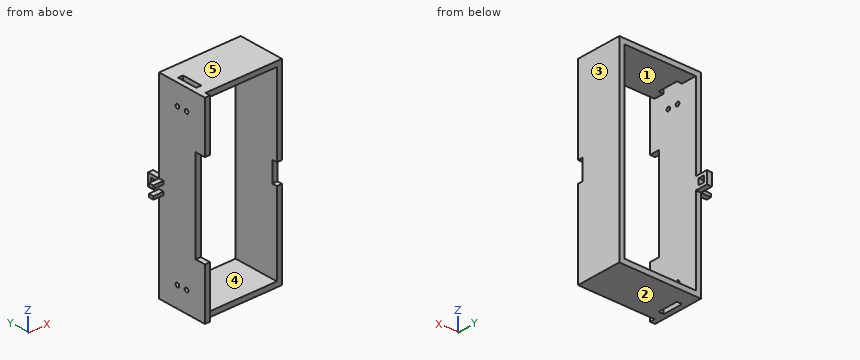
Autodesk Inventor part; units mm, degrees
ref_plane "YZ Plane" through (0, 0, 0) normal (1, 0, 0) x (0, 1, 0)
ref_plane "XZ Plane" through (0, 0, 0) normal (0, 1, 0) x (-1, 0, 0)
ref_plane "XY Plane" through (0, 0, 0) normal (0, 0, 1) x (1, 0, 0)
sketch "Sketch1" plane through (0, 0, 0) normal (1, 0, 0) x (0, 1, 0)
  line L0 (0, 0) -> (50, 0)
  line L1 (50, 0) -> (50, -50)
  line L2 (0, 0) -> (10, 0)
  line L3 (10, -50) -> (0, -50)
  line L4 (0, -50) -> (0, 0)
  line L5 (50, -50) -> (50, -190)
  line L6 (50, -190) -> (0, -190)
  line L7 (0, -190) -> (0, -140)
  line L8 (0, -140) -> (10, -140)
  line L9 (10, -140) -> (10, -50)
  line L10 (0, -105) -> (50, -105) construction
  line L11 (50, -89) -> (62, -89)
  line L12 (62, -89) -> (62, -101)
  line L13 (62, -101) -> (50, -101)
  line L14 (50, -101) -> (50, -89)
  line L15 (59, -92) -> (53, -92)
  line L16 (53, -92) -> (53, -98)
  line L17 (53, -98) -> (59, -98)
  line L18 (59, -98) -> (59, -92)
  point P0 (50, -101)
  dimension "d0" = 50
  dimension "d4" = 50
  dimension "d5" = 10
  dimension "d8" = 190
  dimension "d9" = 50
  dimension "d10" = 12
  dimension "d11" = 12
  dimension "d12" = 3
  dimension "d19" = 89
extrude "Extrusion1" add sketch "Sketch1" along normal blind 5
sketch "Sketch2" plane through (0, 0, 0) normal (-1, 0, 0) x (0, 0, 1)
  line L0 (-190, 50) -> (-101, 50)
  line L1 (-101, 50) -> (-89, 50)
  line L2 (-89, 50) -> (-89, 45)
  line L3 (-89, 45) -> (-101, 45)
  line L4 (-101, 45) -> (-101, 50)
  point P0 (0, 0)
  dimension "d13" = 5
extrude "Extrusion2" add sketch "Sketch2" along normal blind 10
sketch "Sketch3" plane through (0, 50, -89) normal (0, 1, 0) x (1, 0, 0)
  line L0 (-10, 12) -> (-10, 0)
  line L1 (0, 0) -> (0, 12)
  line L2 (-10, 3) -> (0, 3)
  line L3 (0, 3) -> (0, 9)
  line L4 (0, 9) -> (-10, 9)
  line L5 (-10, 9) -> (-10, 3)
  point P0 (0, -89)
  point P1 (-10, 9)
  point P2 (0, 3)
  dimension "d16" = 6
extrude "Extrusion3" cut sketch "Sketch3" against normal blind 10
sketch "Sketch4" plane through (5, 0, 0) normal (1, 0, 0) x (0, 0, -1)
  line L0 (89, 50) -> (0, 50)
  line L1 (0, 0) -> (50, 0)
  line L2 (190, 50) -> (101, 50)
  line L3 (0, 50) -> (5, 50)
  line L4 (5, 50) -> (5, 5)
  line L5 (5, 5) -> (0, 5)
  line L6 (0, 5) -> (0, 50)
  line L7 (190, 0) -> (190, 50)
  line L8 (185, 50) -> (190, 50)
  line L9 (190, 50) -> (190, 5)
  line L10 (190, 5) -> (185, 5)
  line L11 (185, 5) -> (185, 50)
  point P0 (5, 0)
  dimension "d27" = 5
  dimension "d28" = 45
  dimension "d32" = 45
extrude "Extrusion4" add sketch "Sketch4" along normal blind 75
sketch "Sketch6" plane through (0, 0, 0) normal (0, 0, 1) x (1, 0, 0)
  point P0 (0, 0)
sketch "Sketch7" plane through (5, 5, -185) normal (0, 0, 1) x (1, 0, 0)
  line L0 (0, 45) -> (75, 45)
  line L1 (0, 0) -> (75, 0)
  line L2 (75, 45) -> (70, 45)
  line L3 (70, 45) -> (70, 0)
  line L4 (70, 0) -> (75, 0)
  line L5 (75, 0) -> (75, 45)
  point P0 (-5, -5)
  dimension "d29" = 5
extrude "Extrusion6" add sketch "Sketch7" along normal blind 180
sketch "Sketch8" plane through (80, 0, 0) normal (1, 0, 0) x (0, 0, -1)
  line L0 (50, 10) -> (140, 10)
  line L1 (85, 5) -> (105, 5)
  line L2 (105, 5) -> (105, 10)
  line L3 (105, 10) -> (85, 10)
  line L4 (85, 10) -> (85, 5)
  point P0 (0, 0)
  dimension "d33" = 20
extrude "Extrusion7" cut sketch "Sketch8" against normal blind 180
sketch "Sketch9" plane through (5, 0, 0) normal (1, 0, 0) x (0, 0, -1)
  circle A0 centre (20, 30) radius 2
  circle A1 centre (20, 20) radius 2
  circle A2 centre (170, 30) radius 2
  circle A3 centre (170, 20) radius 2
  line L0 (0, 50) -> (0, 5)
  line L1 (190, 5) -> (190, 50)
  line L2 (89, 50) -> (5, 50)
  line L3 (185, 50) -> (101, 50)
  point P0 (0, 0)
  dimension "d36" = 4
  dimension "d37" = 4
  dimension "d38" = 4
  dimension "d39" = 4
  dimension "d40" = 20
  dimension "d41" = 20
  dimension "d42" = 20
  dimension "d43" = 20
  dimension "d44" = 10
  dimension "d45" = 10
  dimension "d46" = 20
  dimension "d47" = 20
extrude "Extrusion8" cut sketch "Sketch9" against normal blind 180
sketch "Sketch10" plane through (0, 0, -190) normal (0, 0, -1) x (-1, 0, 0)
  line L0 (-5, 50) -> (-5, 5)
  line L1 (-5, 15) -> (-10, 15)
  line L2 (-10, 15) -> (-10, 35)
  line L3 (-10, 35) -> (-5, 35)
  line L4 (-5, 35) -> (-5, 15)
  point P0 (0, 0)
  dimension "d50" = 5
  dimension "d51" = 20
extrude "Extrusion9" cut sketch "Sketch10" against normal through all
properties part number "cover"
Model file for the job. Use its own axes, mm. Face numbers are marked on the shaded views. A direction names the side the tool comes from. Coordinates: 2 decimals unless noted, no trailing zeros. Order: outer loops, then holes, each group sorted by start corner. A loop starts at its lowest first (then second) coordinate and runs counter-clockwise, first axis right, second up. Notation, with made-up numbers: (89.5, 47.25) - (138.5, 47.25) arc R8 cw to (138.5, 58.25) - close; hole circle Ø8 at (56.25, -20). An arc over 180 degrees is marked (long way). Return JSON: item names as keys, results as strings. Group by question number.
1) Saw through at A-A, the plane z = -20. Write the cut outline in (x, y), plus the area to 3 significant figures.
2) Saw through at C-C, the plane z = -55. Write the cut outline in (x, y).
3) Tool access for the marked faces 4 and 5: list every direction of +Z, -Z, +X, -X, +Y, -Y with a clear straight run to the whole face (end or side of a thin tool).
4) Saw through at D-D, the plane y = 41.5. Write the cut outline in (x, z).
5) Flat gauge pins, fed straight in: P1, Ø1.5, axis at x = 17, y = 19.5, coming from the +Z side; P2, Ø5.5, axis at x = -4.5, y = 48, coming from the -Z side; P3, Ø3.5, axis at x = -5.5, z = -100, coming from the -Y side; P4, Ø2.5, axis at x = -6, y = 48, coming from the +Z side. Where does each tip first touch, or does it go through?
6) Saw through at B-B, the plane x = 12. Write the cut outline in (y, z), plus the area to 3 significant figures.
7) Mould opens along X. For the marked faces 1, 2 and 3 say: released by +X, released by -X, zero draft, split by the parting line, or undercut.
8) Probe line 1 (Y direction, x = 2, z = -170); line 2 (X direction, y = 26.5, z = -113.5); line 3 (Z direction, x = 19.5, y = 12.5). List the from-to ranges inside material, lowest first. Write a range as from..to.
Values found:
{
 "1": {"outline": "(0, 0) - (5, 0) - (5, 18) - (0, 18) - close; (0, 22) - (5, 22) - (5, 28) - (0, 28) - close; (0, 32) - (5, 32) - (5, 50) - (0, 50) - close; (75, 5) - (80, 5) - (80, 50) - (75, 50) - close", "area": "435 mm²"},
 "2": {"outline": "(0, 10) - (5, 10) - (5, 50) - (0, 50) - close; (75, 5) - (80, 5) - (80, 50) - (75, 50) - close"},
 "3": {"face 4": "+Y, -Y", "face 5": "+Z, +X, -X, +Y, -Y"},
 "4": {"outline": "(0, -190) - (80, -190) - (80, 0) - (0, 0) - close; hole (5, -185) - (75, -185) - (75, -5) - (5, -5) - close"},
 "5": {"P1": "stops at z = 0", "P2": "stops at z = -101", "P3": "stops at y = 45", "P4": "stops at z = -89"},
 "6": {"outline": "(5, -190) - (50, -190) - (50, -185) - (5, -185) - close; (5, -5) - (50, -5) - (50, 0) - (5, 0) - close", "area": "450 mm²"},
 "7": {"face 1": "undercut", "face 2": "zero draft", "face 3": "released by +X"},
 "8": {"line 1": "y = 0..18, 22..28, 32..50", "line 2": "x = 0..5, 75..80", "line 3": "z = -190..-185, -5..0"}
}
